from build123d import *

# Parameters (mm, degrees)
SKETCH1_R           = 1.5
BOSS_EXTRUDE1_DEPTH = 2
SKETCH2_R           = 3
BOSS_EXTRUDE2_DEPTH = 5


with BuildPart() as part:
    # Sketch1 → Boss-Extrude1 (new body)
    with BuildSketch(Plane.XY):
        with BuildLine():
            Line((4.62962963, 4.62962963), (25, 3))
            ThreePointArc((25, 3), (28, 0), (25, -3))
            Line((25, -3), (4.62962963, -4.62962963))
            Line((4.62962963, -4.62962963), (3, -25))
            ThreePointArc((3, -25), (0, -28), (-3, -25))
            Line((-3, -25), (-4.62962963, -4.62962963))
            Line((-4.62962963, -4.62962963), (-25, -3))
            ThreePointArc((-25, -3), (-28, 0), (-25, 3))
            Line((-25, 3), (-4.611543086, 4.855711421))
            Line((-4.611543086, 4.855711421), (-3, 25))
            ThreePointArc((-3, 25), (0, 28), (3, 25))
            Line((3, 25), (4.62962963, 4.62962963))
        make_face()
        with Locations((0, 25)):
            Circle(SKETCH1_R, mode=Mode.SUBTRACT)
        with Locations((25, 0)):
            Circle(SKETCH1_R, mode=Mode.SUBTRACT)
        with Locations((0, -25)):
            Circle(SKETCH1_R, mode=Mode.SUBTRACT)
        with Locations((-25, 0)):
            Circle(SKETCH1_R, mode=Mode.SUBTRACT)
    extrude(amount=BOSS_EXTRUDE1_DEPTH)

    # Sketch2 → Boss-Extrude2 (add)
    with BuildSketch(Plane.XY.offset(2)):
        Circle(SKETCH2_R)
    extrude(amount=BOSS_EXTRUDE2_DEPTH)


solid = part.part
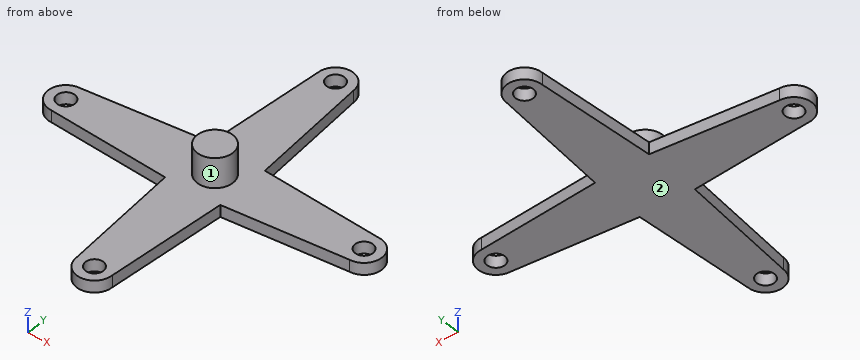
Geometry: final body of the model. Coordinates: model frame, mm. Face numbers are marked on the shaded views. A direction names the side the tool comes from. Coordinates: 2 decimals unless noted, no trailing zeros. Loops run counter-clockwise (first coordinate to the right, second up) from the corner with the lowest first, then second, coordinate; pieces in that order, holes last. Notation, with made-up numbers: (-14.5, 84.5) - (11.5, 84.5) arc R24 ccw to (11.5, 120.5) - close; hole circle Ø5 at (65.5, 87). An arc over 180 degrees is marked (long way). One line per question, with ' | ' between items. Start each with the question number.
(1) Ray query, L1, parallel to Y at x = 0, z = 0.5; L2, parallel to Y at x = 25, z = 0.6; L3, parallel to Z at x = -0.5, y = 13. Return the intervals inside material, ascending. Write a range as from..to.
(2) Cut plane C-C on x = 20.5. Output: boundary loops of the cut face in (y, z), and give its area (3 significant figures).
(3) Reachability of the marked faces 1 and 2 from +Z, -Z, +X, -X, +Y, -Y: full face, straight path, thin tool, end or side. Return the list, or none.
(4) Cut plane A-A on y = 0. Output: boundary loops of the cut face in (x, z).
(5) Cut plane D-D on z = 2.75. Output: boundary loops of the cut face in (x, y), and give its area (3 significant figures).
Here are the results:
1) L1: -28..-26.5, -23.5..23.5, 26.5..28 | L2: -3..-1.5, 1.5..3 | L3: 0..2
2) outline: (-3.36, 0) - (3.36, 0) - (3.36, 2) - (-3.36, 2) - close | area: 13.4 mm²
3) face 1: +Z | face 2: -Z, +X, -X, +Y, -Y
4) outline: (-28, 0) - (-26.5, 0) - (-26.5, 2) - (-28, 2) - close; (-23.5, 0) - (23.5, 0) - (23.5, 2) - (3, 2) - (3, 7) - (-3, 7) - (-3, 2) - (-23.5, 2) - close; (26.5, 0) - (28, 0) - (28, 2) - (26.5, 2) - close
5) outline: circle Ø6 at (0, 0) | area: 28.3 mm²
